from build123d import *

# Parameters (mm, degrees)
SKETCH2_W                 = 85
SKETCH2_H                 = 70
BOSS_EXTRUDE1_DEPTH       = 12
SKETCH4_R                 = 10
CUT_EXTRUDE3_DEPTH        = 10
FILLET2_R                 = 2
M3X0_5_TAPPED_HOLE1_D     = 2.5
M3X0_5_TAPPED_HOLE1_DEPTH = 10
M3X0_5_TAPPED_HOLE1_TIP   = 0.751075774
CUT_EXTRUDE4_DEPTH        = 8


with BuildPart() as part:
    # Sketch2 → Boss-Extrude1 (new body)
    with BuildSketch(Plane(origin=(0, 0, 0), x_dir=(1, 0, 0), z_dir=(0, 1, 0))):
        Rectangle(SKETCH2_W, SKETCH2_H)
    extrude(amount=BOSS_EXTRUDE1_DEPTH)

    # Sketch4 → Cut-Extrude3 (cut)
    with BuildSketch(Plane(origin=(0, 12, 0), x_dir=(1, 0, 0), z_dir=(0, 1, 0))):
        with Locations((42.5, -35)):
            Circle(SKETCH4_R)
        with Locations((-42.5, -35)):
            Circle(SKETCH4_R)
        with Locations((-42.5, 35)):
            Circle(SKETCH4_R)
        with Locations((42.5, 35)):
            Circle(SKETCH4_R)
    extrude(amount=-CUT_EXTRUDE3_DEPTH, mode=Mode.SUBTRACT)

    # Fillet2
    fillet2_edges = [part.edges().sort_by_distance(p)[0] for p in [
        (42.5, 12, 0),
        (0, 12, -35),
        (-42.5, 12, 0),
        (0, 12, 35),
        (35.428932188, 12, -27.928932188),
        (-35.428932188, 12, -27.928932188),
        (-35.428932188, 12, 27.928932188),
        (35.428932188, 12, 27.928932188),
    ]]
    fillet(fillet2_edges, radius=FILLET2_R)

    # M3x0.5 Tapped Hole1
    with Locations(Plane(origin=(0, 2, 0), x_dir=(1, 0, 0), z_dir=(0, 1, 0))):
        with Locations((-39, 31.5), (-39, -31.5), (39, -31.5), (39, 31.5)):
            Hole(M3X0_5_TAPPED_HOLE1_D / 2, depth=M3X0_5_TAPPED_HOLE1_DEPTH)
            with Locations((0, 0, -(M3X0_5_TAPPED_HOLE1_DEPTH + M3X0_5_TAPPED_HOLE1_TIP / 2))):  # 118° drill point
                Cone(0, M3X0_5_TAPPED_HOLE1_D / 2, M3X0_5_TAPPED_HOLE1_TIP, mode=Mode.SUBTRACT)

    # Sketch8 → Cut-Extrude4 (cut)
    with BuildSketch(Plane.XZ):
        with BuildLine():
            Line((35.5, -25), (35.5, 25))
            ThreePointArc((35.5, 25), (34.914213562, 26.414213562), (33.5, 27))
            Line((33.5, 27), (-33.5, 27))
            ThreePointArc((-33.5, 27), (-34.914213562, 26.414213562), (-35.5, 25))
            Line((-35.5, 25), (-35.5, -25))
            ThreePointArc((-35.5, -25), (-34.914213562, -26.414213562), (-33.5, -27))
            Line((-33.5, -27), (33.5, -27))
            ThreePointArc((33.5, -27), (34.914213562, -26.414213562), (35.5, -25))
        make_face()
    extrude(amount=-CUT_EXTRUDE4_DEPTH, mode=Mode.SUBTRACT)


solid = part.part
Here's how the part is built. I have some questions about the finished solid (model axes, mm). A direction names the side the tool comes from. Give positions to 0.01 mm unless a question says otherwise; leave off trailing zeros. Order: outer loops, then holes, each group sorted by start corner. A loop starts at its lowest first (then second) coordinate and runs counter-clockwise, first axis right, second up. Notation, with made-up numbers: (54, 2) -> (104, 2) arc R15 ccw to (104, 8) -> close; hole circle Ø6 at (-31, 38). An arc over 180 degrees is marked (long way). One line per item, written item: value. Start each with the question number.
1. I need wall thicknesses on probe 1 along Z at (x, y) = (-39, 0.7); probe 2 along X at (y, z) = (1.1, -31.5); probe 3 along X at (y, z) = (4.5, 2). Which ranges of each line are inside material? Lowest first, please. Write a range as from..to.
2. Will these pins go through, and if not, where does the flat tip stop? pin 1 Ø3 at (x, z) = (40, 29) entering from +Y; pin 2 Ø4 at (x, z) = (-0.5, -25.5) entering from -Y; pin 3 Ø11 at (x, z) = (-39.5, 31) entering from +Y; pin 4 Ø2 at (x, z) = (16.5, -13.5) entering from -Y.
3. We'd pull the mould along X, two halves only. Please class faces 4 (the face through (-34.93, 3.94, -26.4)), 5 (the face through (-41.93, 11.4, -0.35)), 6 (the face through (41.9, 11.43, -0.35)): released by +X, released by -X, zero draft, split by the parting line, or undercut.
4. Imagine slicing it at B-B, the plane x = -1. List the corners of the cut face in (y, z) for me.
5. For faces 1 (the face through (-37.6, 2, -31.2)), 2 (the face through (-35.5, 4, 0)), 3 (the face through (35.51, 6.06, 27.85)), which set-ups out of +Z, -Z, +X, -X, +Y, -Y let a thin tool reach every point of the face, with its end or its side?
6. Imagine slicing it at C-C, the plane z = -9.5. List the corners of the cut face in (x, y) for me, plus the area to 3 significant figures.
7. Imagine slicing it at A-A, the plane y = 5.5. List the corners of the cut face in (x, z) for me.
8. Imagine slicing it at D-D, the plane x = 39. Count the separate pieces of the cut face and the enclosed holes in it, plus the area to 3 significant figures.
Values follow:
1. probe 1: z = -35..-32.75, -30.25..30.25, 32.75..35
1. probe 2: x = -42.5..-40.25, -37.75..37.75, 40.25..42.5
1. probe 3: x = -42.5..-35.5, 35.5..42.5
2. pin 1: stops at y = 2
2. pin 2: stops at y = 0
2. pin 3: stops at y = 11.32
2. pin 4: stops at y = 8
3. face 4: undercut
3. face 5: released by -X
3. face 6: released by +X
4. outline: (0, -35) -> (10, -35) arc R2 ccw to (12, -33) -> (12, 33) arc R2 ccw to (10, 35) -> (0, 35) -> (0, 27) -> (8, 27) -> (8, -27) -> (0, -27) -> close
5. face 1: -Z, -X, +Y
5. face 2: -Y
5. face 3: +Z, +X, +Y
6. outline: (-42.5, 0) -> (-35.5, 0) -> (-35.5, 8) -> (35.5, 8) -> (35.5, 0) -> (42.5, 0) -> (42.5, 10) arc R2 ccw to (40.5, 12) -> (-40.5, 12) arc R2 ccw to (-42.5, 10) -> close
6. area: 450 mm2
7. outline: (-42.5, -25) arc R10 cw to (-32.5, -35) -> (32.5, -35) arc R10 cw to (42.5, -25) -> (42.5, 25) arc R10 cw to (32.5, 35) -> (-32.5, 35) arc R10 cw to (-42.5, 25) -> close; hole (-35.5, -25) arc R2 ccw to (-33.5, -27) -> (33.5, -27) arc R2 ccw to (35.5, -25) -> (35.5, 25) arc R2 ccw to (33.5, 27) -> (-33.5, 27) arc R2 ccw to (-35.5, 25) -> close
8. separate pieces: 3
8. enclosed holes: 0
8. area: 641 mm2
